The listing builds one solid part. Answer for the finished solid, in the listing's coordinates (mm). Face numbers are marked on the shaded views. A direction names the side the tool comes from. Round coordinates to 2 decimals unless told otherwise and drop trailing zeros. Loops run counter-clockwise (first coordinate to the right, second up) from the corner with the lowest first, then second, coordinate; pieces in that order, holes last. Notation, with made-up numbers: (0, 4.5) -> (13, 4.5) arc R22 ccw to (13, 34.5) -> close; hole circle Ø10 at (27, 46). An arc over 180 degrees is marked (long way). One line per question, with ' | ' between items.
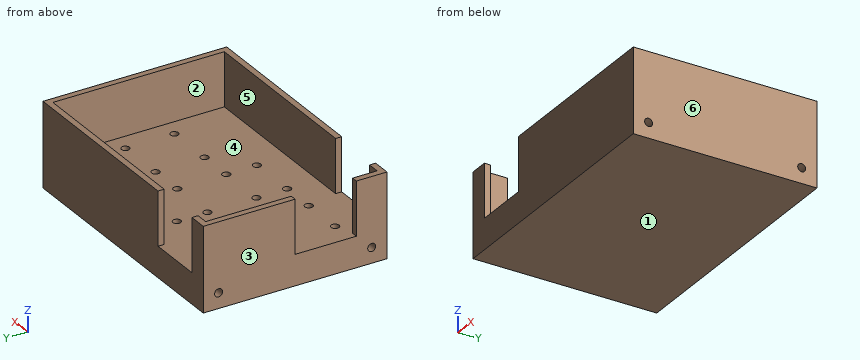
from build123d import *

# Parameters (mm, degrees)
SKETCH1_W          = 76.2
SKETCH1_H          = 107.95
BASE_DEPTH         = 12.7
SKETCH3_W          = 107.95
SKETCH3_H          = 76.2
SKETCH3_W_2        = 102.87
SKETCH3_H_2        = 71.12
WALLS_DEPTH        = 22.225
CUT_EXTRUDE1_DEPTH = 22.225
SKETCH2_R          = 1.650000002
CUT_EXTRUDE2_DEPTH = 6.99999997
SKETCH6_R          = 1.650000002
CUT_EXTRUDE3_DEPTH = 6.99999997
SKETCH7_R          = 1.650000002
CUT_EXTRUDE4_DEPTH = 6.99999997


with BuildPart() as part:
    # Sketch1 → BASE (new body)
    with BuildSketch(Plane(origin=(0, 0, 0), x_dir=(0, 1, 0), z_dir=(0, 0, 1))):
        Rectangle(SKETCH1_W, SKETCH1_H)
    extrude(amount=BASE_DEPTH)

    # Sketch3 → WALLS (add)
    with BuildSketch(Plane.XY.offset(12.7)):
        Rectangle(SKETCH3_W, SKETCH3_H)
        Rectangle(SKETCH3_W_2, SKETCH3_H_2, mode=Mode.SUBTRACT)
    extrude(amount=WALLS_DEPTH)

    # Sketch4 → Cut-Extrude1 (cut)
    with BuildSketch(Plane.XY.offset(34.925)):
        Polygon((-46.355, 38.1), (-23.495, 38.1), (-23.495, -38.1), (-46.355, -38.1), (-46.355, -25.4), (-53.975, -25.4), (-53.975, 0), (-46.355, 0), align=None)
    extrude(amount=-CUT_EXTRUDE1_DEPTH, mode=Mode.SUBTRACT)

    # Sketch2 → Cut-Extrude2 (cut)
    with BuildSketch(Plane.XY.offset(12.7)):
        with Locations((-43.815, 22.86)):
            Circle(SKETCH2_R)
        with Locations((-26.035, 22.86)):
            Circle(SKETCH2_R)
        with Locations((-43.815, -22.86)):
            Circle(SKETCH2_R)
        with Locations((-26.035, -22.86)):
            Circle(SKETCH2_R)
        with Locations((-11.43, -22.86)):
            Circle(SKETCH2_R)
        with Locations((-11.43, -10.16)):
            Circle(SKETCH2_R)
        with Locations((8.89, -10.16)):
            Circle(SKETCH2_R)
        with Locations((8.89, -22.86)):
            Circle(SKETCH2_R)
        with Locations((23.495, -10.16)):
            Circle(SKETCH2_R)
        with Locations((43.815, -10.16)):
            Circle(SKETCH2_R)
        with Locations((43.815, 10.16)):
            Circle(SKETCH2_R)
        with Locations((23.495, 10.16)):
            Circle(SKETCH2_R)
        with Locations((-11.43, 10.16)):
            Circle(SKETCH2_R)
        with Locations((8.89, 22.86)):
            Circle(SKETCH2_R)
        with Locations((-11.43, 22.86)):
            Circle(SKETCH2_R)
        with Locations((8.89, 10.16)):
            Circle(SKETCH2_R)
    extrude(amount=-CUT_EXTRUDE2_DEPTH, mode=Mode.SUBTRACT)

    # Sketch6 → Cut-Extrude3 (cut)
    with BuildSketch(Plane(origin=(-53.975, 0, 0), x_dir=(0, -1, 0), z_dir=(-1, 0, 0))):
        with Locations((-31.75, 6.35)):
            Circle(SKETCH6_R)
        with Locations((31.75, 6.35)):
            Circle(SKETCH6_R)
    extrude(amount=-CUT_EXTRUDE3_DEPTH, mode=Mode.SUBTRACT)

    # Sketch7 → Cut-Extrude4 (cut)
    with BuildSketch(Plane.YZ.offset(53.975)):
        with Locations((-31.75, 6.35)):
            Circle(SKETCH7_R)
        with Locations((31.75, 6.35)):
            Circle(SKETCH7_R)
    extrude(amount=-CUT_EXTRUDE4_DEPTH, mode=Mode.SUBTRACT)


solid = part.part
Q1. Given pin 1 Ø2.5 at (x, y) = (-11.43, -10.16) entering from +Z; pin 2 Ø3.5 at (x, y) = (23, 10) entering from +Z; pin 3 Ø1 at (y, z) = (-32, 6) entering from -X (3 decimals), each flat-ended and moving along its own axis, determine where each tip first touches the part or whether it passes through.
Numbers:
pin 1: z = 5.7 | pin 2: z = 12.7 | pin 3: x = -46.975
Q2. A cutting plane is placed at D-D on x = -17.5. Give the vertices of the cut face in (y, z) (3 decimals).
Numbers:
outline: (-38.1, 0) -> (38.1, 0) -> (38.1, 34.925) -> (35.56, 34.925) -> (35.56, 12.7) -> (-35.56, 12.7) -> (-35.56, 34.925) -> (-38.1, 34.925) -> close
Q3. A cutting plane is placed at B-B on y = 31.75. Give the vertices of the cut face in (x, z) (3 decimals), plus the area to 3 significant figures.
Numbers:
outline: (-53.975, 0) -> (53.975, 0) -> (53.975, 4.7) -> (46.975, 4.7) -> (46.975, 8) -> (53.975, 8) -> (53.975, 34.925) -> (51.435, 34.925) -> (51.435, 12.7) -> (-51.435, 12.7) -> (-51.435, 34.925) -> (-53.975, 34.925) -> (-53.975, 8) -> (-46.975, 8) -> (-46.975, 4.7) -> (-53.975, 4.7) -> close | area: 1,440 mm^2
Q4. A cutting plane is placed at C-C on z = 25. Give the vertices of the cut face in (x, y) (3 decimals), plus the area to 3 significant figures.
Numbers:
outline: (-53.975, -38.1) -> (-46.355, -38.1) -> (-46.355, -35.56) -> (-51.435, -35.56) -> (-51.435, -25.4) -> (-53.975, -25.4) -> close; (-53.975, 0) -> (-51.435, 0) -> (-51.435, 35.56) -> (-46.355, 35.56) -> (-46.355, 38.1) -> (-53.975, 38.1) -> close; (-23.495, -38.1) -> (53.975, -38.1) -> (53.975, 38.1) -> (-23.495, 38.1) -> (-23.495, 35.56) -> (51.435, 35.56) -> (51.435, -35.56) -> (-23.495, -35.56) -> close | area: 729 mm^2
Q5. For a pull along X with two mould halves and no side action, classify the marked faces 1, 2, 3 and 4 as pulls with the +X half, pulls with the -X half, needs draft (parallel to the pull), parting line crosses it, or undercut.
Numbers:
face 1: needs draft | face 2: undercut | face 3: pulls with the -X half | face 4: undercut
Q6. Find the intervals of material crossed by line 1 (Y direction, x = -11.43, z = 9.25); line 2 (X direction, y = 28, z = 33) (3 decimals); line 3 (Y direction, x = -17, z = 27), in increasing order. Write a range as from..to.
Numbers:
line 1: -38.1..-24.51, -21.21..-11.81, -8.51..8.51, 11.81..21.21, 24.51..38.1 | line 2: -53.975..-51.435, 51.435..53.975 | line 3: -38.1..-35.56, 35.56..38.1
Q7. For the marked faces 5 and 6, determine the directions among +Z, -Z, +X, -X, +Y, -Y from which every point of the face is accessible in a straight line to the end or side of a thin tool.
Numbers:
face 5: +Z | face 6: +Z, -Z, +X, +Y, -Y
Q8. A cutting plane is placed at A-A on z = 10.5. Give the number of separate pieces and of enclosed holes in the cut face, plus the area to 3 significant figures.
Numbers:
separate pieces: 1 | enclosed holes: 16 | area: 8,090 mm^2
